For this review, take the finished solid that the model builds, in its own axes (mm). A direction names the side the tool comes from. Round coordinates to 2 decimals unless told otherwise and drop trailing zeros. Write each loop counter-clockwise with the first axis right and the second up, starting at its lowest first coordinate (ties: lowest second). Pieces come first, ordered by that corner, then holes. Notation, with made-up numbers: (70, 21.5) -> (125, 21.5) arc R17 cw to (125, 49.5) -> close; hole circle Ø2 at (6, 46). An arc over 180 degrees is marked (long way). Answer in a Markdown table with one row per item.
from build123d import *

# Parameters (mm, degrees)
FASE1_SIZE = 0.5
FASE2_SIZE = 0.1


with BuildPart() as part:
    # Skizze1 → Rotation1 (revolve)
    with BuildSketch(Plane.XY, mode=Mode.PRIVATE) as rotation1_sk:
        Polygon((-7.5, 2.5), (-6.5, 2.5), (-6.5, 5), (-1.5, 5), (-1.5, 4), (1.5, 4), (1.5, 5), (6.5, 5), (6.5, 2.5), (7.5, 2.5), (7.5, 0.65), (-7.5, 0.65), align=None)
    revolve(rotation1_sk.sketch.rotate(Axis((-7.5, 0, 0), (1, 0, 0)), 90), axis=Axis((-7.5, 0, 0), (1, 0, 0)))

    # Fase1
    fase1_edges = [part.edges().sort_by_distance(p)[0] for p in [
        (6.5, 0, -2.5),
        (1.5, 0, -4),
        (-1.5, 0, -4),
        (-6.5, 0, -2.5),
    ]]
    chamfer(fase1_edges, length=FASE1_SIZE)

    # Fase2
    fase2_edges = [part.edges().sort_by_distance(p)[0] for p in [
        (6.5, 0, -5),
        (1.5, 0, -5),
        (-1.5, 0, -5),
        (-6.5, 0, -5),
    ]]
    chamfer(fase2_edges, length=FASE2_SIZE)


solid = part.part
1) Clearance check with flat-ended pins moving along their axes: pin 1 Ø2 at (y, z) = (2.5, -3.5) entering from +X; pin 2 Ø1.5 at (x, y) = (0.5, -1) entering from +Z; pin 3 Ø1 at (x, z) = (4.5, -2) entering from +Y; pin 4 Ø1 at (y, z) = (0, 0) entering from -X. State where each tip first meets the part, or that it passes through.
Solved:
| item | result |
|---|---|
| pin 1 | x = 6.5 |
| pin 2 | z = 4.15 |
| pin 3 | y = 4.77 |
| pin 4 | through |
2) Consider section A-A on x = 5.25. State the section outline as (y, z) points.
Solved:
| item | result |
|---|---|
| outline | circle Ø10 at (0, 0); hole circle Ø1.3 at (0, 0) |
3) For line 1 (Y direction, x = -5.75, z = 0); line 2 (X direction, y = 3, z = -2.5); line 3 (X direction, y = -2.75, z = 4), list the stretches that pass through material, from the lowest coordinate up. Write a range as [from, to].
Solved:
| item | result |
|---|---|
| line 1 | [-5, -0.65], [0.65, 5] |
| line 2 | [-6.5, 6.5] |
| line 3 | [-6.5, -1.5], [1.5, 6.5] |
4) For faces 4 (the cylindrical face through (4, 0, -5)), 5 (the cylindrical face through (-7.2, -0.1, -2.5)), list the 3-axis set-ups (+Z, -Z, +X, -X, +Y, -Y) from which the entire face can be reached by the end or side of a thin tool; tool diameter is ignored.
Solved:
| item | result |
|---|---|
| face 4 | +X, -X |
| face 5 | -X |
5) Mouldability with a two-part tool opening along X and no side actions: class faces 1 (the flat face through (-7.5, 1, -1)), 2 (the cylindrical face through (0.014, 3.905, -0.867)), 3 (the cylindrical face through (-4, 0, -5)) as pulls with the +X half, pulls with the -X half, needs draft (parallel to the pull), parting line crosses it, or undercut.
Solved:
| item | result |
|---|---|
| face 1 | pulls with the -X half |
| face 2 | undercut |
| face 3 | needs draft |
